Input: part model. Units: mm. Frame: model coordinates. Face numbers are marked on the shaded views. A direction names the side the tool comes from. Round coordinates to 2 decimals unless told otherwise and drop trailing zeros. Order: outer loops, then holes, each group sorted by start corner. A loop starts at its lowest first (then second) coordinate and runs counter-clockwise, first axis right, second up.
Item 1: First-contact query: pin 1 (5 mm diameter, centred on x = 72, z = -4, fed in from +Y); pin 2 (6.5 mm diameter, centred on y = 180, z = 0, fed in from +X). Flat tips, straight axial feed; report the tip coordinate or a pass-through.
Item 2: Cut plane C-C on x = 130.5. Output: boundary loops of the cut face in (y, z).
Item 3: Reachability of the marked faces 1 and 2 from +Z, -Z, +X, -X, +Y, -Y: full face, straight path, thin tool, end or side. Return the list, or none.
Item 4: Cut plane B-B on y = 200. Give the number of separate pieces and of enclosed holes in the cut face, then the cut area to 3 significant figures.
Item 5: Cut plane D-D on y = 107. Output: boundary loops of the cut face in (x, z), then the cut area to 3 significant figures.
Item 6: Line query: L1, parallel to Z at x = -50, y = 180; L2, parallel to Y at x = 46.5, z = 0.25; L3, parallel to X at y = 196.25, z = 0. Output: solid intervals per line, ascending.
Item 7: Cut plane A-A on z = 0. Output: boundary loops of the cut face in (x, y).
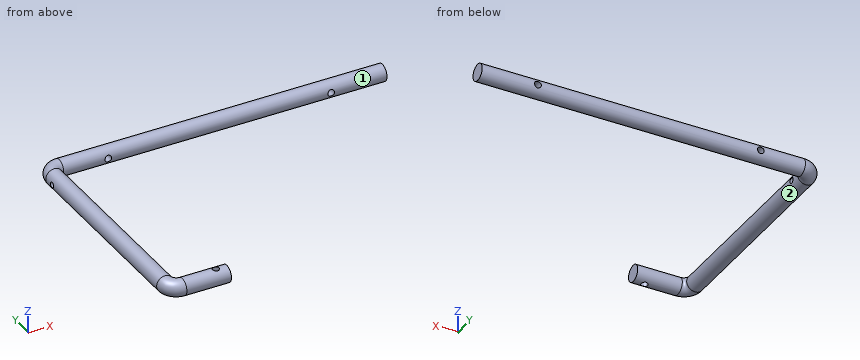
```python
from build123d import *

# Parameters (mm, degrees)
SKETCH_2_R               = 7.5
SKETCH_3_R               = 3
CUT_EXTRUDE_1_DEPTH      = 10
CUT_EXTRUDE_1_DEPTH_BACK = 10
SKETCH_4_R               = 3
CUT_EXTRUDE_2_DEPTH      = 175
SKETCH_5_R               = 2.5
CUT_EXTRUDE_3_DEPTH      = 58.5000001


with BuildPart() as part:
    # Sweep 1: sweep along a path in Sketch 1
    with BuildLine(Plane.XY) as sweep_1_path:
        Line((0, 0), (-40, 0))
        ThreePointArc((-40, 0), (-47.071067812, 2.928932188), (-50, 10))
        Line((-50, 10), (-50, 190))
        ThreePointArc((-50, 190), (-47.071067812, 197.071067812), (-40, 200))
        Line((-40, 200), (250, 200))
    # Sketch 2 → Sweep 1 (sweep)
    with BuildSketch(Plane(origin=(0, 0, 0), x_dir=(0, 0, -1), z_dir=(1, 0, 0))):
        Circle(SKETCH_2_R)
    sweep(path=sweep_1_path.line)

    # Sketch 3 → Cut-Extrude 1 (cut, two sides)
    with BuildSketch(Plane.XY) as cut_extrude_1_sk:
        with Locations((-10, 0)):
            Circle(SKETCH_3_R)
    extrude(amount=CUT_EXTRUDE_1_DEPTH, mode=Mode.SUBTRACT)
    extrude(cut_extrude_1_sk.sketch, amount=-CUT_EXTRUDE_1_DEPTH_BACK, mode=Mode.SUBTRACT)

    # Sketch 4 → Cut-Extrude 2 (cut)
    with BuildSketch(Plane(origin=(0, 50, 0), x_dir=(1, 0, 0), z_dir=(0, 1, 0))):
        with Locations((200, 0)):
            Circle(SKETCH_4_R)
        Circle(SKETCH_4_R)
    extrude(amount=CUT_EXTRUDE_2_DEPTH, mode=Mode.SUBTRACT)

    # Sketch 5 → Cut-Extrude 3 (cut, through all)
    with BuildSketch(Plane(origin=(0, 0, 0), x_dir=(0, 0, -1), z_dir=(1, 0, 0))):
        with Locations((0, 180)):
            Circle(SKETCH_5_R)
    extrude(amount=-CUT_EXTRUDE_3_DEPTH, mode=Mode.SUBTRACT)


solid = part.part
```
From the geometry:
1. pin 1: stops at y = 207.35
1. pin 2: stops at x = -42.5
2. outline: circle Ø15 at (200, 0)
3. face 1: +X
3. face 2: none
4. separate pieces: 1
4. enclosed holes: 2
4. area: 4,480 mm2
5. outline: circle Ø15 at (-50, 0)
5. area: 177 mm2
6. L1: z = -7.5 to -2.5, 2.5 to 7.5
6. L2: y = 192.5 to 207.5
6. L3: x = -56.35 to -3, 3 to 197, 203 to 250
7. outline: (-57.5, 10) arc R17.5 ccw to (-40, -7.5) - (0, -7.5) - (0, 7.5) - (-40, 7.5) arc R2.5 cw to (-42.5, 10) - (-42.5, 177.5) - (-57.5, 177.5) - close; (-57.5, 182.5) - (-42.5, 182.5) - (-42.5, 190) arc R2.5 cw to (-40, 192.5) - (-3, 192.5) - (-3, 207.5) - (-40, 207.5) arc R17.5 ccw to (-57.5, 190) - close; (3, 192.5) - (197, 192.5) - (197, 207.5) - (3, 207.5) - close; (203, 192.5) - (250, 192.5) - (250, 207.5) - (203, 207.5) - close; hole circle Ø6 at (-10, 0)
